Geometry check sheet. Reference: the model listing, model coordinates, mm. A direction names the side the tool comes from. Give positions to 0.01 mm unless a question says otherwise; leave off trailing zeros. Loops run counter-clockwise (first coordinate to the right, second up) from the corner with the lowest first, then second, coordinate; pieces in that order, holes last. Notation, with made-up numbers: (-13, -5) -> (22, -5) arc R28 ccw to (22, 32) -> close; hole circle Ø8 at (3.5, 64). An arc over 180 degrees is marked (long way). Answer in a Markdown table with one row per item. Add a question column.
```python
from build123d import *

# Parameters (mm, degrees)
TUBE_R              = 6.35
BOSS_EXTRUDE1_DEPTH = 9.525
FLANGE_R            = 7.9375
BOSS_EXTRUDE2_DEPTH = 1.5875
SHAFT_R             = 4.7625
CUT_EXTRUDE1_DEPTH  = 9.5875


with BuildPart() as part:
    # tube → Boss-Extrude1 (new body)
    with BuildSketch(Plane(origin=(0, 0, 0), x_dir=(1, 0, 0), z_dir=(0, 1, 0))):
        Circle(TUBE_R)
    extrude(amount=BOSS_EXTRUDE1_DEPTH)

    # Flange → Boss-Extrude2 (add)
    with BuildSketch(Plane(origin=(0, 0, 0), x_dir=(1, 0, 0), z_dir=(0, 1, 0))):
        Circle(FLANGE_R)
    extrude(amount=BOSS_EXTRUDE2_DEPTH)

    # shaft → Cut-Extrude1 (cut)
    with BuildSketch(Plane(origin=(0, 0, 0), x_dir=(1, 0, 0), z_dir=(0, 1, 0))):
        Circle(SHAFT_R)
    extrude(amount=CUT_EXTRUDE1_DEPTH, mode=Mode.SUBTRACT)


solid = part.part
```
1. Sectioned sample at C-C (x = 5.5). Enter the section's corners in (y, z) (1 decimal).
2. Access from +Z, -Z, +X, -X, +Y, -Y to the whole of each face (thin tool, end or side, straight path). Record for faces 1 (the face through (-1.38, 5.5, 6.2)), 2 (the face through (1, 9.525, -5)).
3. Release check for a two-part mould opening along X. For faces 3 (the face through (0, 1.588, -7)), 4 (the face through (-3.78, 4.7, 2.9)), 5 (the face through (-1.72, 0.78, 7.75)) record: released by +X, released by -X, zero draft, split by the parting line, or undercut.
4. Gauge pin test, flat ends, axial feed: pin 1 Ø1.5 at (y, z) = (4.5, -4) entering from +X; pin 2 Ø1.5 at (x, y) = (4.5, 2) entering from -Z; pin 3 Ø1 at (y, z) = (5.5, 4.5) entering from -X. Record the tip position at first contact, or that the pin passes through.
5. Material ranges on L1, parallel to X at y = 7.5, z = 0; L2, parallel to Y at x = 7.25, z = 1, recorded low to high. Write a range as from..to.
Response:
| question | item | result |
|---|---|---|
| 1 | outline | (0, -5.7) -> (1.6, -5.7) -> (1.6, -3.2) -> (9.5, -3.2) -> (9.5, 3.2) -> (1.6, 3.2) -> (1.6, 5.7) -> (0, 5.7) -> close |
| 2 | face 1 | +Y |
| 2 | face 2 | +Z, -Z, +X, -X, +Y |
| 3 | face 3 | zero draft |
| 3 | face 4 | undercut |
| 3 | face 5 | split by the parting line |
| 4 | pin 1 | stops at x = 5.46 |
| 4 | pin 2 | stops at z = -6.93 |
| 4 | pin 3 | stops at x = -4.93 |
| 5 | L1 | x = -6.35..-4.76, 4.76..6.35 |
| 5 | L2 | y = 0..1.59 |
